Here's the drawing with two shaded views (mm, measured from the low corner). I have some questions. A direction names the side the tool comes from. Round coordinates to 2 decimals unless told otherwise and drop trailing zeros. Write each loop counter-clockwise with the first axis right and the second up, starting at its lowest first coordinate (ties: lowest second). Pieces come first, ordered by that corner, then holes. Notation, with made-up numbers: (51.5, -18.5) - (108.5, -18.5) arc R33 ccw to (108.5, 18.5) - close; hole circle Ø9 at (57.5, -39.5). An arc over 180 degrees is marked (long way). Return JSON: item names as keys, results as strings. Group by question number.
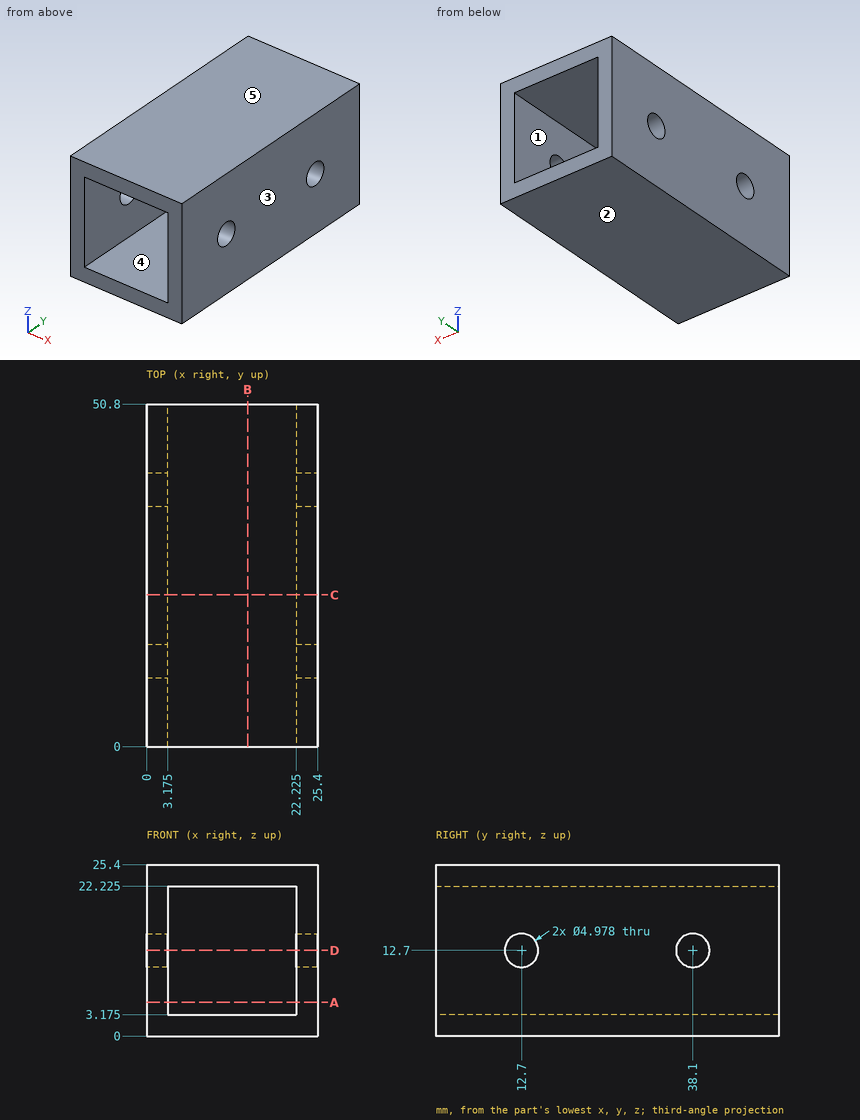
1) Imagine slicing it at D-D (z = 12.7). Please give me the cut outline in (x, y) (1 decimal).
2) Imagine slicing it at B-B (x = 15). Please give me the cut outline in (y, z) (1 decimal).
3) Imagine slicing it at A-A (z = 5). Please give me the cut outline in (x, y) (1 decimal).
4) I need wall thicknesses on line 1 along Y through (x, z) = (1.55, 12.7); line 2 along X through (y, z) = (21.5, 8.25) (1 decimal). Which ranges of each line are inside material? Lowest first, please.
5) If we mould it in two halves opening along Z, with no side actions, what happens to the marked faces 1, 2 and 3? For each: released by +Z, released by -Z, zero draft, split by the parting line, or undercut.
6) For the marked faces 4 and 5, which set-ups out of +Z, -Z, +X, -X, +Y, -Y let a thin tool reach every point of the face, with its end or its side?
7) Imagine slicing it at C-C (y = 22.5). Please give me the cut outline in (x, z) (1 decimal), plus the area to 3 significant figures.
Results found:
{
 "1": {"outline": "(0, 0) - (3.2, 0) - (3.2, 10.2) - (0, 10.2) - close; (0, 15.2) - (3.2, 15.2) - (3.2, 35.6) - (0, 35.6) - close; (0, 40.6) - (3.2, 40.6) - (3.2, 50.8) - (0, 50.8) - close; (22.2, 0) - (25.4, 0) - (25.4, 10.2) - (22.2, 10.2) - close; (22.2, 15.2) - (25.4, 15.2) - (25.4, 35.6) - (22.2, 35.6) - close; (22.2, 40.6) - (25.4, 40.6) - (25.4, 50.8) - (22.2, 50.8) - close"},
 "2": {"outline": "(0, 0) - (50.8, 0) - (50.8, 3.2) - (0, 3.2) - close; (0, 22.2) - (50.8, 22.2) - (50.8, 25.4) - (0, 25.4) - close"},
 "3": {"outline": "(0, 0) - (3.2, 0) - (3.2, 50.8) - (0, 50.8) - close; (22.2, 0) - (25.4, 0) - (25.4, 50.8) - (22.2, 50.8) - close"},
 "4": {"line 1": "y = 0 to 10.21, 15.19 to 35.61, 40.59 to 50.8", "line 2": "x = 0 to 3.2, 22.2 to 25.4"},
 "5": {"face 1": "undercut", "face 2": "released by -Z", "face 3": "zero draft"},
 "6": {"face 4": "+Y, -Y", "face 5": "+Z, +X, -X, +Y, -Y"},
 "7": {"outline": "(0, 0) - (25.4, 0) - (25.4, 25.4) - (0, 25.4) - close; hole (3.2, 3.2) - (22.2, 3.2) - (22.2, 22.2) - (3.2, 22.2) - close", "area": "282 mm²"}
}
